Verification items for the finished model (mm, model axes). Give positions to 0.01 mm unless a question says otherwise; leave off trailing zeros. Order: outer loops, then holes, each group sorted by start corner. A loop starts at its lowest first (then second) coordinate and runs counter-clockwise, first axis right, second up. Notation, with made-up numbers: (45.25, 18) - (61.25, 18) arc R25 cw to (61.25, 46) - close; hole circle Ø4 at (-12.75, -40). An arc over 180 degrees is marked (long way). Answer as a JSON object with one key per item and string values. Group by question number.
(1) Section check B-B (y = -43.5). Record the boundary of the cut face in (x, z), then the cut area to 3 significant figures.
(2) Depth check by flat-ended pin: pin 1 Ø3 at (x, z) = (-106, -51.5) entering from +Y; pin 2 Ø8 at (x, y) = (-68.5, -26) entering from -Z; pin 3 Ø12 at (x, y) = (4.5, -47.5) entering from -Z; pin 4 Ø5 at (y, z) = (-9, -37) entering from +X. Enter the tip coordinate at first touch or a pass-through.
(3) Section check A-A (y = -8.5). Record the boundary of the cut face in (x, z).
(4) Thickness scan on line 1 (Y direction, x = 51.5, z = 9); line 2 (Z direction, x = -31, y = -47); line 3 (X direction, y = -51, z = 60.5). Record the ranges inside material, lowest first.
```python
from build123d import *

# Parameters (mm, degrees)
F0_R     = 120
F0_R_2   = 10
F1_DEPTH = 55
F2_R     = 20
F3_SIZE  = 20
F4_R     = 5


with BuildPart() as f1:
    # F0 (on Front) → F1 (new body)
    with BuildSketch(Plane.XZ):
        with Locations((-49.9732643366, 9.9665783346)):
            Circle(F0_R)
        with Locations((-49.9732643366, 9.9665783346)):
            Circle(F0_R_2, mode=Mode.SUBTRACT)
    extrude(amount=F1_DEPTH)

    # F2
    f2_edges = [f1.edges().sort_by_distance(p)[0] for p in [
        (-169.973264, -55, 9.966578),
        (-169.973264, 0, 9.966578),
    ]]
    fillet(f2_edges, radius=F2_R)

    # F3
    f3_edges = [f1.edges().sort_by_distance(p)[0] for p in [
        (-59.973264, -55, 9.966578),
    ]]
    chamfer(f3_edges, length=F3_SIZE)

    # F4
    f4_edges = [f1.edges().sort_by_distance(p)[0] for p in [
        (-79.973264, -55, 9.966578),
        (-149.973264, -55, 9.966578),
    ]]
    fillet(f4_edges, radius=F4_R)


solid = f1.part
```
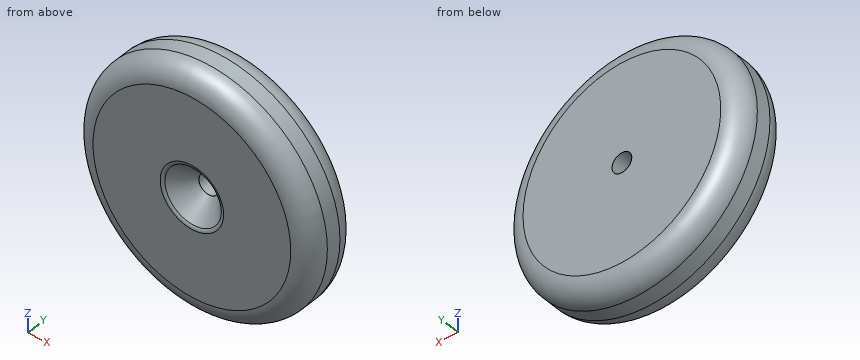
Solutions:
{
 "1": {"outline": "circle Ø236.21 at (-49.97, 9.97); hole circle Ø37 at (-49.97, 9.97)", "area": "42,700 mm2"},
 "2": {"pin 1": "stops at y = 0", "pin 2": "stops at z = -109.15", "pin 3": "stops at z = -97.05", "pin 4": "stops at x = 58.76"},
 "3": {"outline": "circle Ø232.73 at (-49.97, 9.97); hole circle Ø20 at (-49.97, 9.97)"},
 "4": {"line 1": "y = -54.95 to -0.05", "line 2": "z = -104.47 to -1.17, 21.1 to 124.4", "line 3": "x = -149.93 to 49.98"}
}
